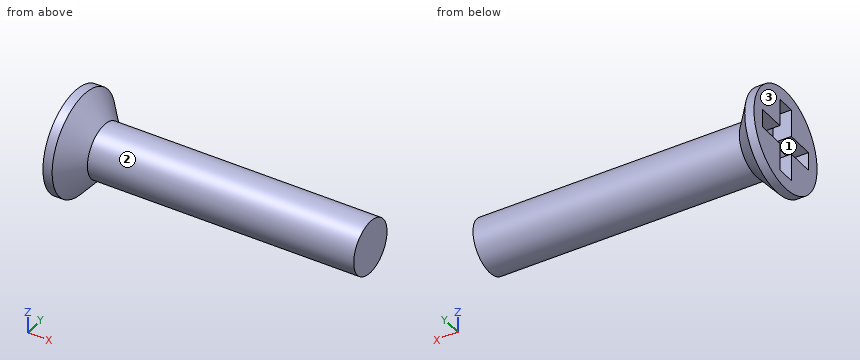
Autodesk Inventor part; units mm, degrees
ref_plane "YZ Plane" through (0, 0, 0) normal (1, 0, 0) x (0, 1, 0)
ref_plane "XZ Plane" through (0, 0, 0) normal (0, 1, 0) x (-1, 0, 0)
ref_plane "XY Plane" through (0, 0, 0) normal (0, 0, 1) x (1, 0, 0)
sketch "Эскиз4" plane through (0, 0, 0) normal (0, 0, 1) x (1, 0, 0)
  line L0 (0, 0) -> (0, 2.75)
  line L1 (1.6, 1.45) -> (16, 1.45)
  line L2 (16, 1.45) -> (16, 0)
  line L3 (16, 0) -> (0, 0)
  line L4 (0, 2.75) -> (0.5, 2.75)
  line L5 (0.5, 2.75) -> (1.6, 1.45)
  dimension "d14" = 16
  dimension "d15" = 1.45
  dimension "d17" = 2.75
  dimension "d18" = 0.5
  dimension "d19" = 1.6
revolve "Вращение1" add sketch "Эскиз4" angle 360 about axis through (16, 0, 0) along (-1, 0, 0)
thread "Резьба2"
sketch "Эскиз5" plane through (0, 0, 0) normal (-1, 0, 0) x (0, 0, 1)
  line L0 (0.5, -2) -> (-0.5, -2)
  line L1 (-0.5, -2) -> (-0.5, 2)
  line L2 (-0.5, 2) -> (0.5, 2)
  line L3 (0.5, 2) -> (0.5, -2)
  line L4 (0.5, -2) -> (-0.5, 2) construction
  line L5 (-0.5, -2) -> (0.5, 2) construction
  line L6 (-2, -0.5) -> (2, -0.5)
  line L7 (2, -0.5) -> (2, 0.5)
  line L8 (2, 0.5) -> (-2, 0.5)
  line L9 (-2, 0.5) -> (-2, -0.5)
  circle A0 centre (0, 0) radius 2.75
  line L10 (-2, -0.5) -> (2, 0.5) construction
  line L11 (2, -0.5) -> (-2, 0.5) construction
  point P0 (-0.5, 0.5)
  point P1 (-0.5, -0.5)
  point P2 (0.5, -0.5)
  point P3 (0.5, 0.5)
  dimension "d23" = 1
  dimension "d24" = 4
extrude "Выдавливание4" cut sketch "Эскиз5" against normal blind 1 contours L0 L1 L6 L3 | L6 L1 L8 L3 | L3 L8 L7 L6 | L6 L9 L8 L1 | L8 L1 L2 L3
properties part number "Болт М3х15"
Source: CAD feature listing. Evaluate the final solid. Frame: model axes, mm. Face numbers are marked on the shaded views. A direction names the side the tool comes from. Coordinates: 2 decimals unless noted, no trailing zeros. Loops run counter-clockwise (first coordinate to the right, second up) from the corner with the lowest first, then second, coordinate; pieces in that order, holes last. Notation, with made-up numbers: (35.5, 89) -> (81.5, 89) arc R34 cw to (81.5, 124) -> close; hole circle Ø10 at (-31, 54). An arc over 180 degrees is marked (long way). One line per item, written item: value. Start each with the question number.
Q1. Section query A-A, the plane z = 0. Return the cut outline in (x, y).
Q2. Set-up query: the marked faces 1, 2 and 3. Return all of +Z, -Z, +X, -X, +Y, -Y with unobstructed straight access to the full face (end or side cutting, diameter ignored); none if empty.
Q3. Contact query for flat-ended pins moving along their axis: P1, Ø1.1, axis at x = 0.5, z = -1, coming from the +Y side; P2, Ø3, axis at x = 8.5, z = 0.5, coming from the -Y side; P3, Ø2, axis at x = 8.5, z = 1, coming from the +Y side. Output: stop coordinate, or through.
Q4. Line query: line 1 along X through (y, z) = (-0.3, -0.4); line 2 along Z through (x, y) = (7.5, -0.1); line 3 along Y through (x, z) = (13.75, -0.4). Output: solid intervals per line, ascending.
Q5. Section query C-C, the plane x = 12. Return the cut outline in (y, z), and give its area (3 significant figures).
Results:
1. outline: (0, -2.75) -> (0.5, -2.75) -> (1.6, -1.45) -> (16, -1.45) -> (16, 1.45) -> (1.6, 1.45) -> (0.5, 2.75) -> (0, 2.75) -> (0, 2) -> (1, 2) -> (1, -2) -> (0, -2) -> close
2. face 1: -X
2. face 2: +X
2. face 3: +Z, -Z, -X, +Y, -Y
3. P1: y = 2.71
3. P2: y = -1.45
3. P3: y = 1.45
4. line 1: 1 to 16
4. line 2: -1.45 to 1.45
4. line 3: -1.39 to 1.39
5. outline: circle Ø2.9 at (0, 0)
5. area: 6.61 mm^2
